```python
from build123d import *

# Parameters (mm, degrees)
SKETCH1_W                = 29
SKETCH1_H                = 40
BOSS_EXTRUDE1_DEPTH      = 20
SKETCH2_W                = 29
SKETCH2_H                = 8
CUT_EXTRUDE1_DEPTH       = 15
SKETCH3_R                = 3.15
CUT_EXTRUDE2_DEPTH       = 30
FILLET1_R                = 17
BOSS_EXTRUDE2_DEPTH      = 2
BOSS_EXTRUDE2_DEPTH_BACK = 32
SKETCH4_R                = 2.3


with BuildPart() as part:
    # Sketch1 → Boss-Extrude1 (new body)
    with BuildSketch(Plane.XY):
        with Locations((14.5, -20)):
            Rectangle(SKETCH1_W, SKETCH1_H)
    extrude(amount=BOSS_EXTRUDE1_DEPTH)

    # Sketch2 → Cut-Extrude1 (cut)
    with BuildSketch(Plane(origin=(0, 0, 0), x_dir=(1, 0, 0), z_dir=(0, 1, 0))):
        with Locations((14.5, -10)):
            Rectangle(SKETCH2_W, SKETCH2_H)
    extrude(amount=-CUT_EXTRUDE1_DEPTH, mode=Mode.SUBTRACT)

    # Sketch3 → Cut-Extrude2 (cut)
    with BuildSketch(Plane.XY.offset(20)):
        with BuildLine():
            Line((0, 0), (0, -15))
            Line((0, -15), (10.60969448, -1.859056995))
            ThreePointArc((10.60969448, -1.859056995), (12.344160839, -0.488641279), (14.5, 0))
            Line((14.5, 0), (0, 0))
        make_face()
        with BuildLine():
            Line((29, 0), (14.5, 0))
            ThreePointArc((14.5, 0), (16.655839161, -0.488641279), (18.39030552, -1.859056995))
            Line((18.39030552, -1.859056995), (29, -15))
            Line((29, -15), (29, 0))
        make_face()
        Polygon((5, -40), (0, -35), (0, -40), align=None)
        Polygon((29, -35), (24, -40), (29, -40), align=None)
        with Locations((14.5, -5)):
            Circle(SKETCH3_R)
    extrude(amount=-CUT_EXTRUDE2_DEPTH, mode=Mode.SUBTRACT)

    # Fillet1
    fillet1_edges = [part.edges().sort_by_distance(p)[0] for p in [
        (29, -35, 10),
        (0, -35, 10),
    ]]
    fillet(fillet1_edges, radius=FILLET1_R)

    # Sketch4 → Boss-Extrude2 (add, two sides: drawn at the far end of the back side and taken through both)
    with BuildSketch(Plane(origin=(29, 0, 0), x_dir=(0, 0, -1), z_dir=(1, 0, 0)).offset(-BOSS_EXTRUDE2_DEPTH_BACK)):
        with Locations(Location((-10, -23, 0), (0, 0, 90))):
            Circle(SKETCH4_R)
    extrude(amount=BOSS_EXTRUDE2_DEPTH + BOSS_EXTRUDE2_DEPTH_BACK)


solid = part.part
```
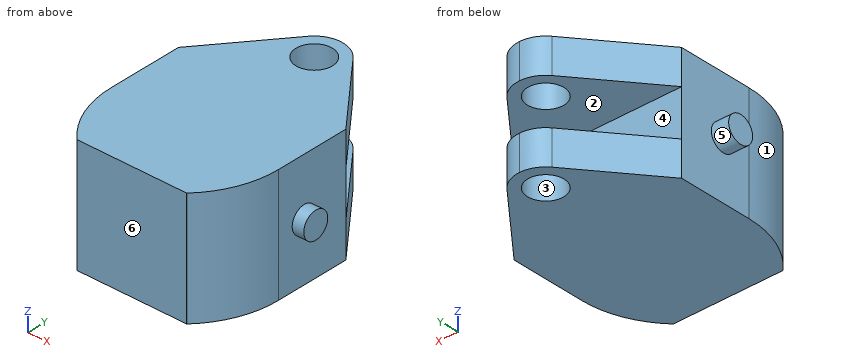
Can you work these out from the model? Positions are in its coordinate system, mm. Face numbers are marked on the shaded views. A direction names the side the tool comes from. Round coordinates to 2 decimals unless told otherwise and drop trailing zeros. Loops run counter-clockwise (first coordinate to the right, second up) from the corner with the lowest first, then second, coordinate; pieces in that order, holes last. Notation, with made-up numbers: (12, 54) -> (17, 54) arc R22 cw to (17, 85) -> close; hole circle Ø11 at (23, -9.5). An arc over 180 degrees is marked (long way). One line per item, written item: value. Start each with the question number.
1. For the marked faces 4, 5 and 6, which set-ups out of +Z, -Z, +X, -X, +Y, -Y let a thin tool reach every point of the face, with its end or its side?
2. If we mould it in two halves opening along Y, with no side actions, what happens to the marked faces 1, 2 and 3? For each: pulls with the +Y half, pulls with the -Y half, needs draft (parallel to the pull), parting line crosses it, or undercut.
3. If we section it at B-B, the plane y = -9: Write out the boundary of the cut face in (x, z), then the cut area to 3 significant figures.
4. If we section it at D-D, the plane y = -5: Write out the boundary of the cut face in (x, z), then the cut area to 3 significant figures.
5. If I drill on probe 1 along Y at (x, z) = (14.5, 16.8); probe 2 along Z at (x, y) = (10.5, -9.5); probe 3 along X at (y, z) = (-24, 7), over which ranges is the centre line in solid material (lowest first)?
6. For pin 1 (6 mm diameter, centred on x = 0.5, z = 8, fed in from -Y); pin 2 (3 mm diameter, centred on y = -35, z = 6, fed in from -X); pin 3 (2 mm diameter, centred on y = -9, z = 3, fed in from +X), each with a flat end and sliding along its axis, tell me the tip position at first contact or that it passes through.
Calculated:
1. face 4: +X, -X, +Y
1. face 5: -X
1. face 6: +Z, -Z, +X, -X, -Y
2. face 1: pulls with the -Y half
2. face 2: needs draft
2. face 3: undercut
3. outline: (4.84, 0) -> (24.16, 0) -> (24.16, 6) -> (4.84, 6) -> close; (4.84, 14) -> (24.16, 14) -> (24.16, 20) -> (4.84, 20) -> close
3. area: 232 mm²
4. outline: (8.07, 0) -> (11.35, 0) -> (11.35, 6) -> (8.07, 6) -> close; (8.07, 14) -> (11.35, 14) -> (11.35, 20) -> (8.07, 20) -> close; (17.65, 0) -> (20.93, 0) -> (20.93, 6) -> (17.65, 6) -> close; (17.65, 14) -> (20.93, 14) -> (20.93, 20) -> (17.65, 20) -> close
4. area: 78.6 mm²
5. probe 1: y = -40 to -8.15, -1.85 to 0
5. probe 2: z = 0 to 6, 14 to 20
5. probe 3: x = 0 to 29
6. pin 1: stops at y = -38.29
6. pin 2: stops at x = 0.93
6. pin 3: stops at x = 24.96
